For this review, take the finished solid that the model builds, in its own axes (mm). A direction names the side the tool comes from. Round coordinates to 2 decimals unless told otherwise and drop trailing zeros. Order: outer loops, then holes, each group sorted by start corner. A loop starts at its lowest first (then second) coordinate and runs counter-clockwise, first axis right, second up. Notation, with made-up numbers: M -35,-32.75 L -5,-32.75 A28 cw -5,-5.75 Z; hole C 83,-8.75 d9. An arc over 180 degrees is marked long. Answer as a JSON object with one key per item and string values.
from build123d import *

# Parameters (mm, degrees)
SKETCH1_R                  = 6.5
BOSS_EXTRUDE1_DEPTH        = 1
BOSS_EXTRUDE2_DEPTH        = 14.5
BOSS_EXTRUDE2_DEPTH_BACK   = 7
M3_TAPPED_HOLE1_AT_2_COUNT = 2
M3_TAPPED_HOLE1_AT_2_PITCH = 78.345788017
M3_TAPPED_HOLE1_AT_3_COUNT = 2
M3_TAPPED_HOLE1_AT_3_PITCH = 36


with BuildPart() as part:
    # Sketch1 → Boss-Extrude1 (new body)
    with BuildSketch(Plane(origin=(0, 0, 0), x_dir=(1, 0, 0), z_dir=(0, 1, 0))):
        with BuildLine():
            Line((11.636363636, 26.548917894), (-9.50963812, 18.294364031))
            ThreePointArc((-9.50963812, 18.294364031), (-14.147260888, 22.497589825), (-18.5, 18))
            Line((-18.5, 18), (-18.5, 12.519984026))
            ThreePointArc((-18.5, 12.519984026), (-9, 0), (-18.5, -12.519984026))
            Line((-18.5, -12.519984026), (-18.5, -18))
            ThreePointArc((-18.5, -18), (-14.147260888, -22.497589825), (-9.50963812, -18.294364031))
            Line((-9.50963812, -18.294364031), (11.636363636, -26.548917894))
            ThreePointArc((11.636363636, -26.548917894), (35.040161132, -25.341748118), (49.626979567, -7))
            Line((49.626979567, -7), (63.125355805, -4.158876316))
            ThreePointArc((63.125355805, -4.158876316), (66.5, 0), (63.125355805, 4.158876316))
            Line((63.125355805, 4.158876316), (49.626979567, 7))
            ThreePointArc((49.626979567, 7), (35.040161132, 25.341748118), (11.636363636, 26.548917894))
        make_face()
        with Locations(Location((0, -8, 0), (0, 0, 270))):
            Circle(SKETCH1_R, mode=Mode.SUBTRACT)
    extrude(amount=BOSS_EXTRUDE1_DEPTH)

    # Sketch2 → Boss-Extrude2 (add, two sides: drawn at the far end of the back side and taken through both)
    with BuildSketch(Plane(origin=(0, 1, 0), x_dir=(1, 0, 0), z_dir=(0, 1, 0)).offset(-BOSS_EXTRUDE2_DEPTH_BACK)):
        Polygon((-11.25, 16.41228676), (-11.25, 19.58771324), (-14, 21.175426481), (-16.75, 19.58771324), (-16.75, 16.41228676), (-14, 14.824573519), align=None)
        Polygon((-14, -14.824573519), (-11.25, -16.41228676), (-11.25, -19.58771324), (-14, -21.175426481), (-16.75, -19.58771324), (-16.75, -16.41228676), align=None)
        Polygon((65, 1.58771324), (62.25, 3.175426481), (59.5, 1.58771324), (59.5, -1.58771324), (62.25, -3.175426481), (65, -1.58771324), align=None)
    extrude(amount=BOSS_EXTRUDE2_DEPTH + BOSS_EXTRUDE2_DEPTH_BACK)

    # Sketch4 → M3 Tapped Hole1 (revolve, cut)
    with BuildSketch(Plane(origin=(-14, 15.5, -18), x_dir=(0, 0, 1), z_dir=(1, 0, 0))):
        Polygon((0, 0), (0, 8.251075774), (1.25, 7.5), (1.25, 0), align=None)
    m3_tapped_hole1 = revolve(axis=Axis((-14, 21.85, -18), (0, -1, 0)), mode=Mode.SUBTRACT)

    # M3 Tapped Hole1 at 2: M3 Tapped Hole1 ×2
    with Locations(*[Vector(0.9732495125772933, 0, 0.22975070460841018) * (i * M3_TAPPED_HOLE1_AT_2_PITCH) for i in range(1, M3_TAPPED_HOLE1_AT_2_COUNT)]):
        add(m3_tapped_hole1, mode=Mode.SUBTRACT)

    # M3 Tapped Hole1 at 3: M3 Tapped Hole1 ×2
    with Locations(*[(0, 0, i * M3_TAPPED_HOLE1_AT_3_PITCH) for i in range(1, M3_TAPPED_HOLE1_AT_3_COUNT)]):
        add(m3_tapped_hole1, mode=Mode.SUBTRACT)

    # Mirror2: M3 Tapped Hole1 across plane
    add(m3_tapped_hole1.mirror(Plane.ZX.offset(4.75)), mode=Mode.SUBTRACT)

    # Mirror2 copy 1 sketch → Mirror2 copy 1 (revolve, cut)
    with BuildSketch(Plane(origin=(62.25, -6, 0), x_dir=(0, 0, 1), z_dir=(1, 0, 0))):
        Polygon((0, 0), (0, -8.251075774), (1.25, -7.5), (1.25, 0), align=None)
    revolve(axis=Axis((62.25, -12.35, 0), (0, -1, 0)), mode=Mode.SUBTRACT)

    # Mirror2 copy 2 sketch → Mirror2 copy 2 (revolve, cut)
    with BuildSketch(Plane(origin=(-14, -6, 18), x_dir=(0, 0, 1), z_dir=(1, 0, 0))):
        Polygon((0, 0), (0, -8.251075774), (1.25, -7.5), (1.25, 0), align=None)
    revolve(axis=Axis((-14, -12.35, 18), (0, -1, 0)), mode=Mode.SUBTRACT)


solid = part.part
1) Add section A-A on y = -2. State the section outline as (x, z) points, and give its area (3 significant figures).
Geometry check:
{"outline": "M -16.75,-19.59 L -14,-21.18 L -11.25,-19.59 L -11.25,-16.41 L -14,-14.82 L -16.75,-16.41 Z; M -16.75,16.41 L -14,14.82 L -11.25,16.41 L -11.25,19.59 L -14,21.18 L -16.75,19.59 Z; M 59.5,-1.59 L 62.25,-3.18 L 65,-1.59 L 65,1.59 L 62.25,3.18 L 59.5,1.59 Z; hole C -14,-18 d2.5; hole C -14,18 d2.5; hole C 62.25,0 d2.5", "area": "63.9 mm²"}
2) Add section C-C on x = 0. State the section outline as (y, z) points.
Geometry check:
{"outline": "M 0,-22.01 L 1,-22.01 L 1,1.5 L 0,1.5 Z; M 0,14.5 L 1,14.5 L 1,22.01 L 0,22.01 Z"}
3) Machinability: for faces 1 (the flat face through (63.644, -3.042, -2.37)), 2 (the flat face through (63.61, 8.15, 2.39)), 3 (the flat face through (-11.25, -3, -18)), 4 (the flat face through (-16.75, 8, 18)), which of the approach directions +Z, -Z, +X, -X, +Y, -Y give a long, thin tool a straight path to every point of the face, cutting with its end or side? Answer none if there is none.
Geometry check:
{"face 1": "-Z, +X, -Y", "face 2": "+Z, +X, +Y", "face 3": "+Z, -Z, +X, -Y", "face 4": "+Z, -Z, -X, +Y"}
4) For L1, parallel to Z at x = -14, y = 13.25; L2, parallel to X at y = 10, z = 18; L3, parallel to X at y = -1.25, z = 0, list the stretches that pass through material, from the lowest coordinate up.
Geometry check:
{"L1": "z = -21.18 to -19.25, -16.75 to -14.82, 14.82 to 16.75, 19.25 to 21.18", "L2": "x = -16.75 to -15.25, -12.75 to -11.25", "L3": "x = 59.5 to 61, 63.5 to 65"}
5) Mouldability with a two-part tool opening along X and no side actions: class faces 5 (the flat face through (-15, -6, -17)), 6 (the cylindrical face through (-14.1, 0.5, -22.5)), 7 (the flat face through (60.856, 8.148, 2.37)), 8 (the conical face through (62.07, 2.12, 0.12)) as +X half, -X half, draft (parallel to the pull), parting line (faces both ways), or undercut.
Geometry check:
{"face 5": "draft", "face 6": "undercut", "face 7": "-X half", "face 8": "undercut"}
6) Insertion check: P1, Ø1, axis at y = 8, z = 17.5, coming from the -X side; P2, Ø1.6, axis at y = -3, z = -17, coming from the +X side; P3, Ø3, axis at x = 42, y = 0.5, coming from the -Z side. Each pin has a flat end and moves straight along its axis. Give the tip position at first contact, or say it passes through.
Geometry check:
{"P1": "stops at x = -16.75", "P2": "stops at x = -11.25", "P3": "stops at z = -21.68"}
7) Add section D-D on y = 5.25. State the section outline as (x, z) points.
Geometry check:
{"outline": "M -16.75,-19.59 L -14,-21.18 L -11.25,-19.59 L -11.25,-16.41 L -14,-14.82 L -16.75,-16.41 Z; M -16.75,16.41 L -14,14.82 L -11.25,16.41 L -11.25,19.59 L -14,21.18 L -16.75,19.59 Z; M 59.5,-1.59 L 62.25,-3.18 L 65,-1.59 L 65,1.59 L 62.25,3.18 L 59.5,1.59 Z"}
8) Add section B-B on z = 5. State the section outline as (x, y) points, and give its area (3 significant figures).
Geometry check:
{"outline": "M -10,0 L -5.77,0 L -5.77,1 L -10,1 Z; M 5.77,0 L 59.13,0 L 59.13,1 L 5.77,1 Z", "area": "57.6 mm²"}
